from build123d import *

# Parameters (mm, degrees)
MAINBODY_DWG_W  = 23.08
MAINBODY_DWG_H  = 40.84
MAIN_BODY_DEPTH = 10
PINS_DWG_W      = 16
PINS_DWG_H      = 1
PINS_DEPTH      = 6
RELIEF_DWG_W    = 10.001117723
RELIEF_DWG_H    = 19
RELIEF_DWG_W_2  = 20
RELIEF_DWG_H_2  = 14
RELIEF_DEPTH    = 7


with BuildPart() as part:
    # MAINBODY_DWG → MAIN_BODY (new body)
    with BuildSketch(Plane(origin=(0, 0, 0), x_dir=(1, 0, 0), z_dir=(0, 1, 0))):
        Rectangle(MAINBODY_DWG_W, MAINBODY_DWG_H)
    extrude(amount=MAIN_BODY_DEPTH)

    # PINS_DWG → PINS (add)
    with BuildSketch(Plane.ZY.offset(11.54)):
        with Locations((11.42, 9.5)):
            Rectangle(PINS_DWG_W, PINS_DWG_H)
    extrude(amount=PINS_DEPTH)

    # RELIEF_DWG → RELIEF (cut)
    with BuildSketch(Plane(origin=(0, 10, 0), x_dir=(1, 0, 0), z_dir=(0, 1, 0))):
        with Locations((6.539441139, 10.92)):
            Rectangle(RELIEF_DWG_W, RELIEF_DWG_H)
        with Locations((1.54, -13.42)):
            Rectangle(RELIEF_DWG_W_2, RELIEF_DWG_H_2)
    extrude(amount=-RELIEF_DEPTH, mode=Mode.SUBTRACT)


solid = part.part
Can you work these out from the model? Positions are in its coordinate system, mm. A direction names the side the tool comes from. Round coordinates to 2 decimals unless told otherwise and drop trailing zeros. Order: outer loops, then holes, each group sorted by start corner. A loop starts at its lowest first (then second) coordinate and runs counter-clockwise, first axis right, second up. Notation, with made-up numbers: (73, -5.75) - (88, -5.75) arc R32 cw to (88, 27.25) - close; hole circle Ø6 at (12, 4.25). An arc over 180 degrees is marked (long way). Answer in a Markdown table with one row per item.
(1) Suppose I cut it at C-C, the plane z = 4.5. Please give me the cut outline in (x, y).
From the geometry:
| item | result |
|---|---|
| outline | (-17.54, 9) - (-11.54, 9) - (-11.54, 0) - (11.54, 0) - (11.54, 10) - (-17.54, 10) - close |
(2) Suppose I cut it at A-A, the plane x = 4. Please give me the cut outline in (y, z), plus the area to 3 significant figures.
From the geometry:
| item | result |
|---|---|
| outline | (0, -20.42) - (3, -20.42) - (3, -1.42) - (10, -1.42) - (10, 6.42) - (3, 6.42) - (3, 20.42) - (0, 20.42) - close |
| area | 177 mm2 |
(3) Which directions (+Z, -Z, +X, -X, +Y, -Y) give clear straight access to the entire face, cutting with the end or side of a thin tool? Please do faces 1 (the face through (-14, 9, 11)), 2 (the face through (1, 7, 6.42)), 3 (the face through (-14.5, 9.5, 3.42)), 4 (the face through (-14.5, 9.5, 19.42)), 5 (the face through (6, 3, -11)).
From the geometry:
| item | result |
|---|---|
| face 1 | +Z, -Z, -X, -Y |
| face 2 | +Z, +X, +Y |
| face 3 | -Z, -X, +Y, -Y |
| face 4 | +Z, -X, +Y, -Y |
| face 5 | -Z, +X, +Y |
(4) Please list where these lines run through material, in increasing order: L1, parallel to Y at x = -11.75, z = 15; L2, parallel to X at y = 9.75, z = 10; L3, parallel to Y at x = 2.5, z = -12.5. Write a range as from..to.
From the geometry:
| item | result |
|---|---|
| L1 | y = 9..10 |
| L2 | x = -17.54..-8.46 |
| L3 | y = 0..3 |
(5) For P1, Ø2, axis at y = 9, z = -7, coming from the +X side; P2, Ø0.5, axis at x = -14, y = 9.5, coming from the -Z side; P3, Ø3, axis at y = 6.5, z = -8.5, coming from the -X side, each with a flat end and sliding along its axis, tell me the tip position at first contact or that it passes through.
From the geometry:
| item | result |
|---|---|
| P1 | stops at x = 1.54 |
| P2 | stops at z = 3.42 |
| P3 | stops at x = -11.54 |
(6) Suppose I cut it at D-D, the plane x = -1.75. Please give me the cut outline in (y, z).
From the geometry:
| item | result |
|---|---|
| outline | (0, -20.42) - (10, -20.42) - (10, 6.42) - (3, 6.42) - (3, 20.42) - (0, 20.42) - close |
(7) Suppose I cut it at B-B, the plane y = 3.75. Please give me the cut outline in (x, z).
From the geometry:
| item | result |
|---|---|
| outline | (-11.54, -20.42) - (1.54, -20.42) - (1.54, -1.42) - (11.54, -1.42) - (11.54, 6.42) - (-8.46, 6.42) - (-8.46, 20.42) - (-11.54, 20.42) - close |
